```python
from build123d import *

# Parameters (mm, degrees)
SKETCH1_R           = 19.05
SKETCH1_R_2         = 14.478
BOSS_EXTRUDE1_DEPTH = 38.1
BOSS_EXTRUDE2_START = -10.16
SKETCH2_R           = 14.478
SKETCH2_R_2         = 6.35
BOSS_EXTRUDE2_DEPTH = 27.94
CUT_EXTRUDE1_DEPTH  = 10.16
CUT_EXTRUDE2_START  = -10.16
SKETCH4_R           = 19.05
SKETCH4_R_2         = 6.35
CUT_EXTRUDE2_DEPTH  = 10.16


with BuildPart() as part:
    # Sketch1 → Boss-Extrude1 (new body)
    with BuildSketch(Plane.XY):
        Circle(SKETCH1_R)
        Circle(SKETCH1_R_2, mode=Mode.SUBTRACT)
    extrude(amount=-BOSS_EXTRUDE1_DEPTH)

    # Sketch2 → Boss-Extrude2 (add)
    with BuildSketch(Plane.XY.offset(BOSS_EXTRUDE2_START)):
        Circle(SKETCH2_R)
        Circle(SKETCH2_R_2, mode=Mode.SUBTRACT)
    extrude(amount=-BOSS_EXTRUDE2_DEPTH)

    # Sketch3 → Cut-Extrude1 (cut)
    with BuildSketch(Plane.XY):
        with BuildLine():
            Line((-5.540490734, 13.375927872), (-7.290119387, 17.599905094))
            ThreePointArc((-7.290119387, 17.599905094), (0, 19.05), (7.290119387, 17.599905094))
            Line((7.290119387, 17.599905094), (5.540490734, 13.375927872))
            ThreePointArc((5.540490734, 13.375927872), (0, 14.478), (-5.540490734, 13.375927872))
        make_face()
        with BuildLine():
            Line((13.375927872, 5.540490734), (17.599905094, 7.290119387))
            ThreePointArc((17.599905094, 7.290119387), (19.05, 0), (17.599905094, -7.290119387))
            Line((17.599905094, -7.290119387), (13.375927872, -5.540490734))
            ThreePointArc((13.375927872, -5.540490734), (14.478, 0), (13.375927872, 5.540490734))
        make_face()
        with BuildLine():
            Line((5.540490734, -13.375927872), (7.290119387, -17.599905094))
            ThreePointArc((7.290119387, -17.599905094), (0, -19.05), (-7.290119387, -17.599905094))
            Line((-7.290119387, -17.599905094), (-5.540490734, -13.375927872))
            ThreePointArc((-5.540490734, -13.375927872), (0, -14.478), (5.540490734, -13.375927872))
        make_face()
        with BuildLine():
            Line((-13.375927872, -5.540490734), (-17.599905094, -7.290119387))
            ThreePointArc((-17.599905094, -7.290119387), (-19.05, 0), (-17.599905094, 7.290119387))
            Line((-17.599905094, 7.290119387), (-13.375927872, 5.540490734))
            ThreePointArc((-13.375927872, 5.540490734), (-14.478, 0), (-13.375927872, -5.540490734))
        make_face()
    extrude(amount=-CUT_EXTRUDE1_DEPTH, mode=Mode.SUBTRACT)

    # Sketch4 → Cut-Extrude2 (cut)
    with BuildSketch(Plane(origin=(0, 0, -38.1), x_dir=(-1, 0, 0), z_dir=(0, 0, -1)).offset(CUT_EXTRUDE2_START)):
        with Locations(Location((0, 0, 0), (0, 0, 157.5))):
            Circle(SKETCH4_R)
        with Locations(Location((0, 0, 0), (0, 0, 180))):
            Circle(SKETCH4_R_2, mode=Mode.SUBTRACT)
    extrude(amount=CUT_EXTRUDE2_DEPTH, mode=Mode.SUBTRACT)


solid = part.part
```
Input: part model. Units: mm. Frame: model coordinates. A direction names the side the tool comes from. Coordinates: 2 decimals unless noted, no trailing zeros. Write each loop counter-clockwise with the first axis right and the second up, starting at its lowest first coordinate (ties: lowest second). Pieces come first, ordered by that corner, then holes. Notation, with made-up numbers: (75, 7) - (81, 7) arc R27 cw to (81, 43) - close; hole circle Ø4 at (23, 1). An arc over 180 degrees is marked (long way). Put each result on its own line as item: value. Start each with the question number.
1) Reachability of faces 1 (the face through (-6.403, 15.458, -5.009)), 2 (the face through (10.294, 10.181, -5.009)), 3 (the face through (-15.52, 6.43, -5.01)) from +Z, -Z, +X, -X, +Y, -Y: full face, straight path, thin tool, end or side. Return the list, or none.
2) Cut plane C-C (z = -25.25). Return the cut outline in (x, y).
3) Ray query, L1, parallel to Y at x = 0, z = -23.25; L2, parallel to Z at x = 10.5, y = 7; L3, parallel to X at y = -4.5, z = -10.25. Return the intervals inside material, ascending.
4) Cut plane D-D (x = -12). Return the cut outline in (y, z).
5) Contact query for flat-ended pins moving along their axis: pin 1 (3 mm diameter, centred on y = -2.5, z = -18, fed in from +X); pin 2 (6 mm diameter, centred on x = -1, z = -8.5, fed in from +Y); pin 3 (2 mm diameter, centred on y = 6, z = -6, fed in from +X). Output: stop coordinate, or through.
6) Cut plane A-A (y = 0). Return the cut outline in (x, z), plus the area to 3 significant figures.
7) Mould query, pull axis X, two halves, no side actions, for faces 4 (the face through (-12, -11, 0)), 5 (the face through (-15.458, -6.403, -5.009)), 6 (the face through (15.52, -6.43, -5.01)), 7 (the face through (-1.38, -6.2, -18.93)). Classes: pulls with the +X half, pulls with the -X half, needs draft (parallel to the pull), parting line crosses it, or undercut.
Resolved:
1. face 1: +Z, +Y
1. face 2: +Z
1. face 3: +Z, -X
2. outline: circle Ø38.1 at (0, 0); hole circle Ø12.7 at (0, 0)
3. L1: y = -19.05 to -6.35, 6.35 to 19.05
3. L2: z = -27.94 to -10.16
3. L3: x = -18.51 to -4.48, 4.48 to 18.51
4. outline: (-14.8, -27.94) - (14.8, -27.94) - (14.8, 0) - (8.1, 0) - (8.1, -10.16) - (-8.1, -10.16) - (-8.1, 0) - (-14.8, 0) - close
5. pin 1: stops at x = 19.02
5. pin 2: stops at y = 19.05
5. pin 3: stops at x = 16.9
6. outline: (-19.05, -27.94) - (-6.35, -27.94) - (-6.35, -10.16) - (-19.05, -10.16) - close; (6.35, -27.94) - (19.05, -27.94) - (19.05, -10.16) - (6.35, -10.16) - close
6. area: 452 mm2
7. face 4: needs draft
7. face 5: pulls with the -X half
7. face 6: pulls with the +X half
7. face 7: undercut
